```python
from build123d import *

# Parameters (mm, degrees)
F0_R     = 8.435
F0_R_2   = 4.625
F1_DEPTH = 2.125
F3_R     = 3.75
F3_R_2   = 2
F4_DEPTH = 14.605
F5_R     = 2
F6_DEPTH = 10.16


# Not quite as in the source:
# - a pattern or mirror of a feature is missing from the dataset's text; its kind, count and spacing are read off the source's solid


with BuildPart() as f1:
    # F0 (on Top) → F1 (new body, symmetric)
    with BuildSketch(Plane.XY):
        Circle(F0_R)
        Circle(F0_R_2, mode=Mode.SUBTRACT)
    extrude(amount=F1_DEPTH, both=True)

    # F3 (on offset) → F4 (join)
    with BuildSketch(Plane.XZ.offset(6.53)):
        Circle(F3_R)
        Circle(F3_R_2, mode=Mode.SUBTRACT)
        Circle(F3_R_2)
    f4 = extrude(amount=F4_DEPTH)

    # F4_copies: F4 across plane
    add(f4.mirror(Plane(origin=(0, 0, 0), x_dir=(-0.2588190451, 0.9659258263, 0), z_dir=(0.9659258263, 0.2588190451, 0))))

    # F5 (on face) → F6 (cut)
    with BuildSketch(Plane.XZ.offset(21.135)):
        Circle(F5_R)
    f6 = extrude(amount=-F6_DEPTH, mode=Mode.SUBTRACT)

    # F6_copies: F6 across plane
    add(f6.mirror(Plane(origin=(0, 0, 0), x_dir=(-0.2588190451, 0.9659258263, 0), z_dir=(0.9659258263, 0.2588190451, 0))), mode=Mode.SUBTRACT)


solid = f1.part
```
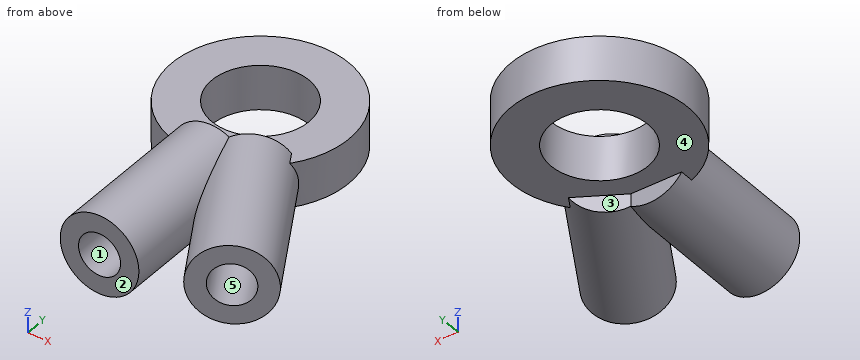
Geometry check sheet. Reference: the model listing, model coordinates, mm. Face numbers are marked on the shaded views. A direction names the side the tool comes from. Coordinates: 2 decimals unless noted, no trailing zeros. Order: outer loops, then holes, each group sorted by start corner. A loop starts at its lowest first (then second) coordinate and runs counter-clockwise, first axis right, second up. Notation, with made-up numbers: M -20.5,-35 L -11.5,-35 A29 ccw -11.5,2 Z; hole C -30.75,68.25 d9. An arc over 180 degrees is marked long. Answer as a JSON object with one key per item and string values.
Q1. Cross-section at A-A on y = 0. Record the cut outline in (x, z) (3 decimals).
Results are:
{"outline": "M -8.435,-2.125 L -4.625,-2.125 L -4.625,2.125 L -8.435,2.125 Z; M 4.625,-2.125 L 8.435,-2.125 L 8.435,2.125 L 4.625,2.125 Z"}
Q2. Tool access check on the marked faces 1 and 2. Record the directions out of +Z, -Z, +X, -X, +Y, -Y that give a thin tool (end or side, any length) a straight path to the whole face; none if there is none.
Results are:
{"face 1": "-Y", "face 2": "+Z, -Z, +X, -X, -Y"}
Q3. Scan lines: line 1 (Y direction, x = 0, z = -1.3) (3 decimals); line 2 (Z direction, x = 0, y = -13.5); line 3 (Z direction, x = 1.5, y = -5.75) (3 decimals). Record each from-to range of solid material in increasing order.
Results are:
{"line 1": "y = -10.975 to -4.625, 4.625 to 8.435", "line 2": "z = -3.75 to -2, 2 to 3.75", "line 3": "z = -2.125 to 2.125"}
Q4. Cross-section at D-D on x = -4.25. Record the cut outline in (y, z) (3 decimals).
Results are:
{"outline": "M -7.286,-2.125 L -1.824,-2.125 L -1.824,2.125 L -7.286,2.125 Z; M 1.824,-2.125 L 7.286,-2.125 L 7.286,2.125 L 1.824,2.125 Z"}
Q5. Depth check by flat-ended pin: pin 1 Ø3 at (y, z) = (-12.5, 3) entering from +X; pin 2 Ø1.3 at (x, z) = (0.5, -3) entering from +Y; pin 3 Ø1.5 at (x, z) = (-4, -2) entering from +Y; pin 4 Ø5 at (x, y) = (-1, -0.5) entering from -Z. Enter the tip coordinate at first touch or a pass-through.
Results are:
{"pin 1": "stops at x = 11.54", "pin 2": "stops at y = -6.53", "pin 3": "stops at y = 7.78", "pin 4": "passes through"}
Q6. Release check for a two-part mould opening along X. For the marked faces 3, 4 and 5 record: released by +X, released by -X, zero draft, split by the parting line, or undercut.
Results are:
{"face 3": "released by -X", "face 4": "zero draft", "face 5": "undercut"}
Q7. Cross-section at B-B on x = 0. Record the cut outline in (y, z) (3 decimals), and give its area (3 significant figures).
Results are:
{"outline": "M -21.135,-3.75 L -6.53,-3.75 L -6.53,-2.125 L -4.625,-2.125 L -4.625,2.125 L -6.53,2.125 L -6.53,3.75 L -21.135,3.75 L -21.135,2 L -10.975,2 L -10.975,-2 L -21.135,-2 Z; M 4.625,-2.125 L 8.435,-2.125 L 8.435,2.125 L 4.625,2.125 Z", "area": "93.2 mm²"}
Q8. Cross-section at C-C on z = 0. Record the cut outline in (x, y) (3 decimals), and give its area (3 significant figures).
Results are:
{"outline": "M -3.75,-21.135 L -2,-21.135 L -2,-10.975 L 2,-10.975 L 2,-21.135 L 3.75,-21.135 L 3.75,-13.995 L 7.32,-20.178 L 8.835,-19.303 L 3.755,-10.505 L 7.22,-8.505 L 12.3,-17.303 L 13.815,-16.428 L 7.025,-4.668 A8.435 ccw long -3.75,-7.556 Z; hole C 0,0 d9.25", "area": "260 mm²"}
